Design review of the part shown in the three views and the two pictorial views. Dimensions are in mm from the part's minimum x, y and z. Coordinates: 2 decimals unless noted, no trailing zeros. Write each loop counter-clockwise with the first axis right and the second up, starting at its lowest first coordinate (ties: lowest second). Pieces come first, ordered by that corner, then holes. Notation, with made-up numbers: (10, -20) -> (57, -20) arc R27 ccw to (57, -3) -> close; hole circle Ø11 at (27.25, 41.5). An arc over 180 degrees is marked (long way). Write each question's results on one line, items separated by ' | '.
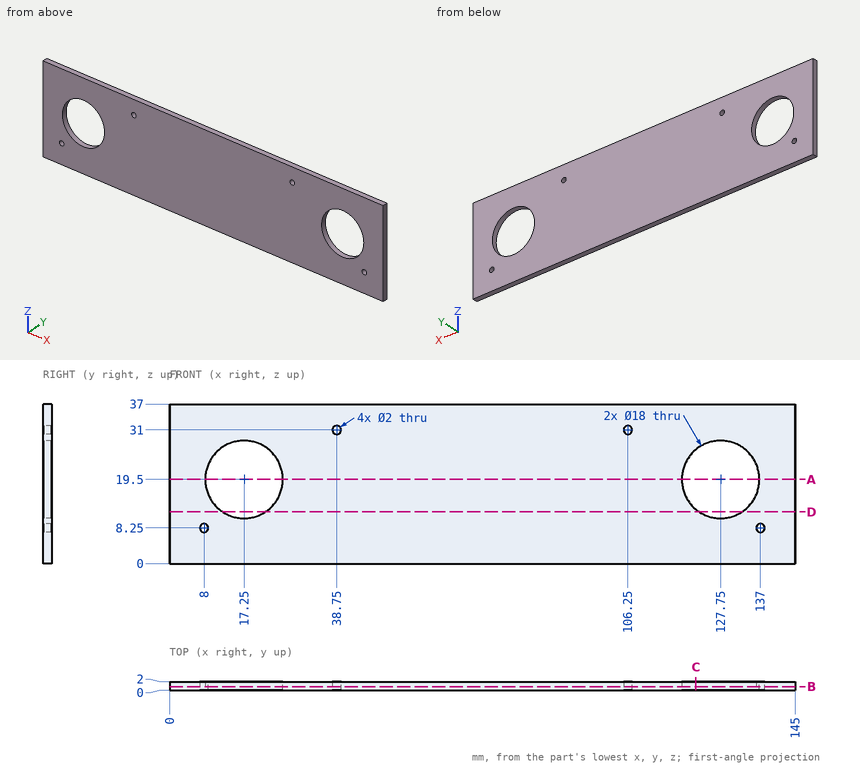
Q1. For line 1 (X direction, y = 1.4, z = 15.5); line 2 (X direction, y = 0.65, z = 9); line 3 (Z direction, x = 38.75, y = 0.5), list the stretches that pass through material, from the lowest coordinate up. Write a range as from..to.
Solution:
line 1: 0..9.19, 25.31..119.69, 135.81..145 | line 2: 0..7.34, 8.66..136.34, 137.66..145 | line 3: 0..30, 32..37
Q2. Add section B-B (y = 0.85). Write out the cut boundary in (x, z), plus the area to 3 significant figures.
Solution:
outline: (0, 0) -> (145, 0) -> (145, 37) -> (0, 37) -> close; hole circle Ø2 at (8, 8.25); hole circle Ø18 at (17.25, 19.5); hole circle Ø2 at (38.75, 31); hole circle Ø2 at (106.25, 31); hole circle Ø18 at (127.75, 19.5); hole circle Ø2 at (137, 8.25) | area: 4,840 mm²
Q3. Clearance check with flat-ended pins moving along their axes: P1, Ø1.8, axis at x = 38.75, z = 31, coming from the +Y side; P2, Ø2, axis at x = 67.5, z = 15, coming from the -Y side. State where each tip first meets the part, or that it passes through.
Solution:
P1: through | P2: y = 0
Q4. Add section D-D (z = 12). Write out the cut boundary in (x, y), plus the area to 3 significant figures.
Solution:
outline: (0, 0) -> (12.28, 0) -> (12.28, 2) -> (0, 2) -> close; (22.22, 0) -> (122.78, 0) -> (122.78, 2) -> (22.22, 2) -> close; (132.72, 0) -> (145, 0) -> (145, 2) -> (132.72, 2) -> close | area: 250 mm²
Q5. Add section C-C (x = 122). Write out the cut boundary in (y, z).
Solution:
outline: (0, 0) -> (2, 0) -> (2, 12.58) -> (0, 12.58) -> close; (0, 26.42) -> (2, 26.42) -> (2, 37) -> (0, 37) -> close
Q6. Add section A-A (z = 19.5). Write out the cut boundary in (x, y), plus the area to 3 significant figures.
Solution:
outline: (0, 0) -> (8.25, 0) -> (8.25, 2) -> (0, 2) -> close; (26.25, 0) -> (118.75, 0) -> (118.75, 2) -> (26.25, 2) -> close; (136.75, 0) -> (145, 0) -> (145, 2) -> (136.75, 2) -> close | area: 218 mm²
